The listing builds one solid part. Answer for the finished solid, in the listing's coordinates (mm). A direction names the side the tool comes from. Coordinates: 2 decimals unless noted, no trailing zeros. Write each loop counter-clockwise with the first axis right and the second up, starting at its lowest first coordinate (ties: lowest second). Pieces come first, ordered by that corner, then holes. Notation, with made-up numbers: M 81,24.25 L 98,24.25 A27 ccw 98,62.25 Z; hole C -33.5,-3.75 d6. An arc over 180 degrees is marked long. Put each result on its own line as item: value. Start each with the question number.
```python
from build123d import *

# Parameters (mm, degrees)
F1_DEPTH = 220
F2_W     = 358.275851
F2_H     = 3
F3_DEPTH = 6


with BuildPart() as f1:
    # F0 (on Front) → F1 (new body)
    with BuildSketch(Plane.XZ):
        Polygon((300, 0), (0, 0), (19, -19), (281, -19), align=None)
    extrude(amount=-F1_DEPTH)

    # F2 (on face) → F3 (cut)
    with BuildSketch(Plane(origin=(0, 0, -19), x_dir=(1, 0, 0), z_dir=(0, 0, -1))):
        with Locations((172.087271, -20.5)):
            Rectangle(F2_W, F2_H)
    extrude(amount=-F3_DEPTH, mode=Mode.SUBTRACT)


solid = f1.part
```
1) Straight lines are drawn through the part: probe 1 along Y at (x, z) = (123.5, -16.75); probe 2 along X at (y, z) = (156.5, -13); probe 3 along X at (y, z) = (192, -3.75). For each, find the intervals that lie inside material, in ascending order.
2) For faces 1 (the face through (148, 220, -9)), 2 (the face through (148, 19, -16)), determine the directions among +Z, -Z, +X, -X, +Y, -Y from which every point of the face is accessible in a straight line to the end or side of a thin tool.
3) Given pin 1 Ø1.5 at (x, y) = (199, 20) entering from -Z; pin 2 Ø1 at (y, z) = (88.5, -12.5) entering from -X; pin 3 Ø4 at (x, y) = (154.5, 80) entering from +Z; pin 4 Ø4 at (y, z) = (102.5, -16) entering from +X, each flat-ended and moving along its own axis, determine where each tip first touches the part or whether it passes through.
4) A cutting plane is placed at B-B on z = -9.5. Write down the section's boundary in (x, y).
5) Determine the mould class of faces 3 (the face through (148, 0, -9)), 4 (the face through (148, 22, -16)), 5 (the face through (148, 120, -19)) for opening direction Y: +Y half, -Y half, draft (parallel to the pull), parting line (faces both ways), or undercut.
6) A cutting plane is placed at A-A on y = 177.5. Write down the section's boundary in (x, z), then the cut area to 3 significant figures.
Answers follow:
1. probe 1: y = 0 to 19, 22 to 220
1. probe 2: x = 13 to 287
1. probe 3: x = 3.75 to 296.25
2. face 1: +Z, -Z, +X, -X, +Y
2. face 2: -Z, +X, -X
3. pin 1: stops at z = -13
3. pin 2: stops at x = 12
3. pin 3: stops at z = 0
3. pin 4: stops at x = 286
4. outline: M 9.5,0 L 290.5,0 L 290.5,220 L 9.5,220 Z
5. face 3: -Y half
5. face 4: undercut
5. face 5: draft
6. outline: M 0,0 L 19,-19 L 281,-19 L 300,0 Z
6. area: 5,340 mm²
